Answer from the drawing. Dimensions are ordinates in mm from the lowest x, y and z of the part. Round coordinates to 2 decimals unless told otherwise and drop trailing zeros. Order: outer loops, then holes, each group sorted by start corner. A loop starts at its lowest first (then second) coordinate and runs counter-clockwise, first axis right, second up. Notation, with made-up numbers: (-37, 61.25) -> (-33, 61.25) arc R28 ccw to (-33, 87.25) -> close; hole circle Ø6 at (-14.75, -34.75). An arc over 180 degrees is marked (long way). Use a Markdown table: item, result. Add a question column.
Item 1: A flat-ended cylindrical pin translates along its axis: P1, Ø5.5, axis at x = 12, z = 12, coming from the -Y side. Find the tip coordinate at first contact, or state that the pin passes through.
Item 2: A cutting plane is placed at A-A, the plane x = 12. Determine the outline of the cut face in (y, z), plus the area to 3 significant figures.
Item 3: A cutting plane is placed at D-D, the plane z = 21.25. Determine the outline of the cut face in (x, y), plus the area to 3 significant figures.
Item 4: For a pull along X with two mould halves and no side action, classify the marked faces 1, 2 and 3 as +X half, -X half, draft (parallel to the pull), parting line (faces both ways), or undercut.
Item 5: A cutting plane is placed at B-B, the plane z = 12. Determine the outline of the cut face in (x, y).
Item 6: A cutting plane is placed at C-C, the plane y = 1.6. Determine the outline of the cut face in (x, z).
Item 7: Find the intervals of material crossed by L1, parallel to Z at x = 12, y = 0.85; L2, parallel to Z at x = 10, y = 0.8; L3, parallel to Z at x = 22.25, y = 0.7, in increasing order. Write a range as [from, to].
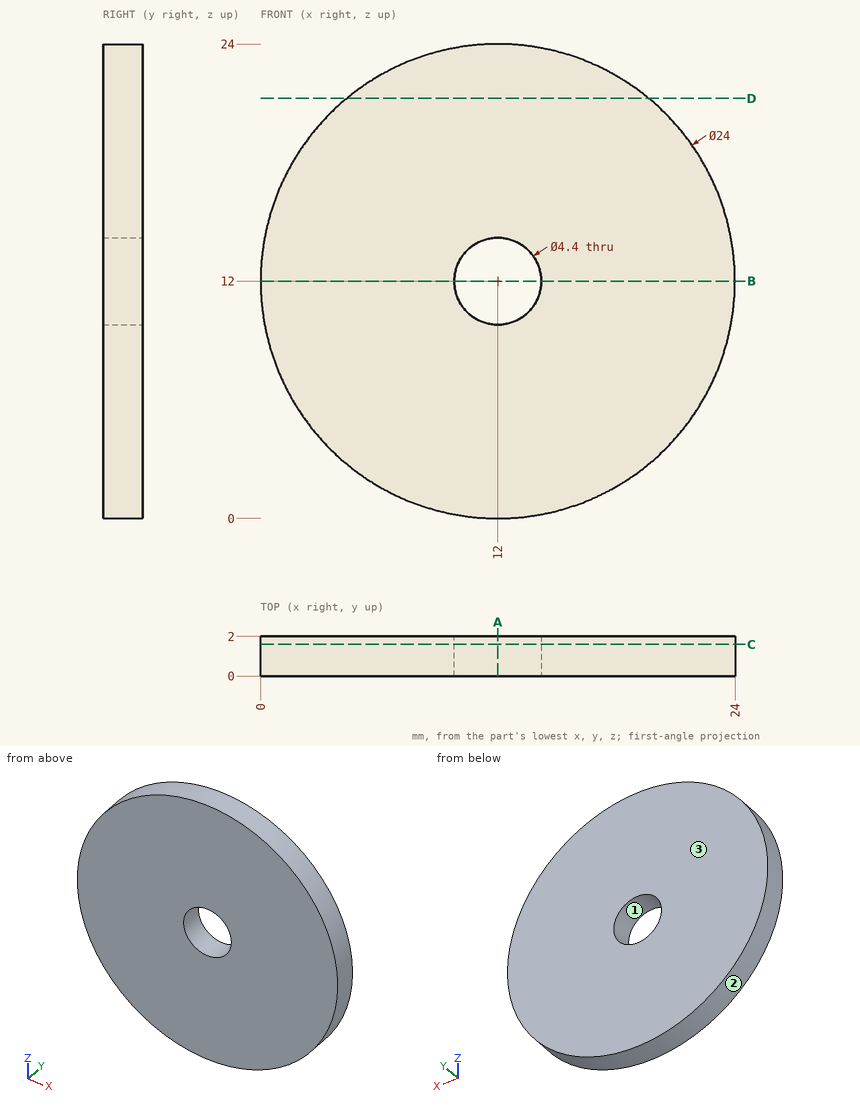
Reported:
| question | item | result |
|---|---|---|
| 1 | P1 | y = 0 |
| 2 | outline | (0, 0) -> (2, 0) -> (2, 9.8) -> (0, 9.8) -> close; (0, 14.2) -> (2, 14.2) -> (2, 24) -> (0, 24) -> close |
| 2 | area | 39.2 mm² |
| 3 | outline | (4.36, 0) -> (19.64, 0) -> (19.64, 2) -> (4.36, 2) -> close |
| 3 | area | 30.6 mm² |
| 4 | face 1 | undercut |
| 4 | face 2 | parting line |
| 4 | face 3 | draft |
| 5 | outline | (0, 0) -> (9.8, 0) -> (9.8, 2) -> (0, 2) -> close; (14.2, 0) -> (24, 0) -> (24, 2) -> (14.2, 2) -> close |
| 6 | outline | circle Ø24 at (12, 12); hole circle Ø4.4 at (12, 12) |
| 7 | L1 | [0, 9.8], [14.2, 24] |
| 7 | L2 | [0.17, 11.08], [12.92, 23.83] |
| 7 | L3 | [5.76, 18.24] |
